Could you check a few things on this drawing? It's one solid part, dimensions in mm from its lowest x, y, z. A direction names the side the tool comes from. Coordinates: 2 decimals unless noted, no trailing zeros. Loops run counter-clockwise (first coordinate to the right, second up) from the corner with the lowest first, then second, coordinate; pieces in that order, holes last.
1) Thinking about a two-plate mould opening in Y: for the marked faces 1, 2 and 3, which applies, released by +Y, released by -Y, zero draft, split by the parting line, or undercut?
2) Imagine slicing it at C-C on y = 3.5. Please give me the cut outline in (x, z), plus the area to 3 significant figures.
3) If I drill on line 1 along Y through (x, z) = (4, 9.25); line 2 along Y through (x, z) = (4, 7.5); line 3 along Y through (x, z) = (4, 11), over which ranges is the centre line in solid material (lowest first)?
4) Imagine slicing it at B-B on x = 4. Please give me the cut outline in (y, z), plus the area to 3 significant figures.
5) Imagine slicing it at A-A on z = 9. Please give me the cut outline in (x, y).
6) Will these pins go through, and if not, where does the flat tip stop? P1, Ø3.5, axis at x = 4, y = 19.5, coming from the -Z side; P2, Ø1.4, axis at x = 4, y = 11, coming from the -Z side; P3, Ø5, axis at y = 9, z = 12, coming from the -X side; P4, Ø1.5, axis at x = 5, z = 6, coming from the -Y side.
7) For the marked faces 4, 5, 6 and 7, which set-ups out of +Z, -Z, +X, -X, +Y, -Y let a thin tool reach every point of the face, with its end or its side?
8) Imagine slicing it at D-D on z = 3.5. Please give me the cut outline in (x, y).
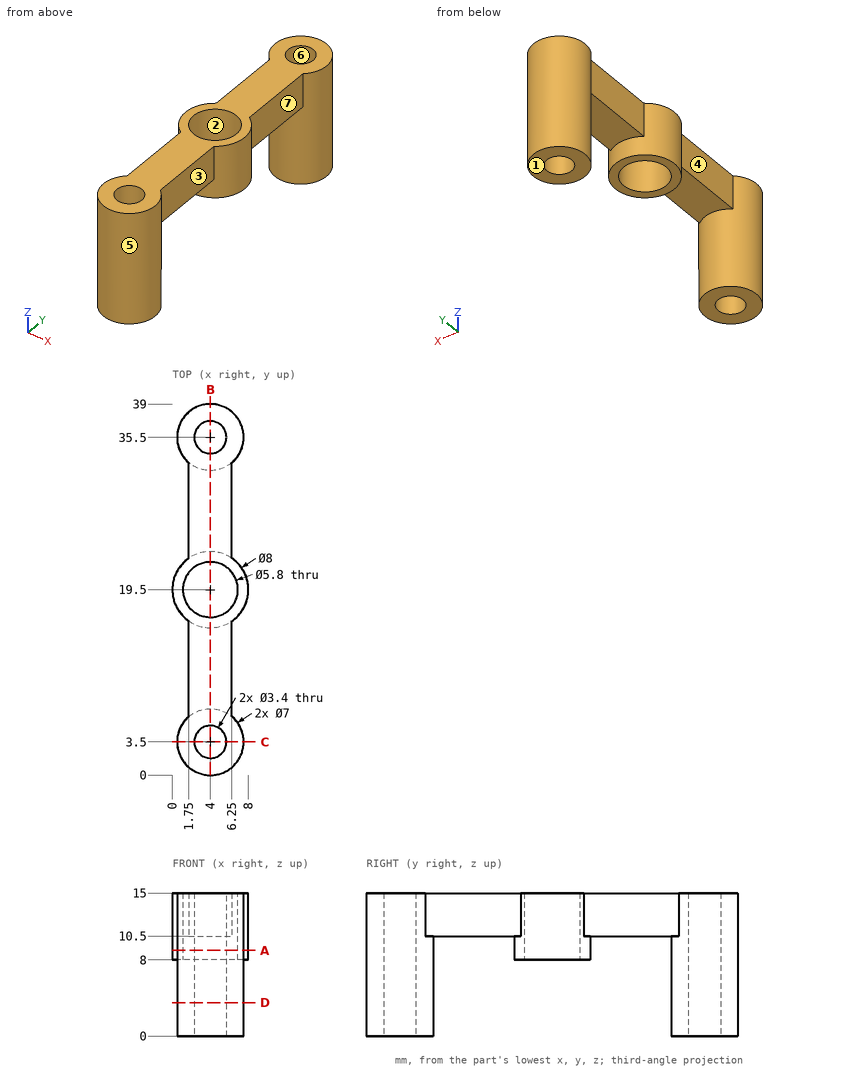
Filled in:
1. face 1: zero draft
1. face 2: undercut
1. face 3: undercut
2. outline: (0.5, 0) - (2.3, 0) - (2.3, 15) - (0.5, 15) - close; (5.7, 0) - (7.5, 0) - (7.5, 15) - (5.7, 15) - close
2. area: 54.0 mm2
3. line 1: y = 0 to 1.8, 5.2 to 7, 15.5 to 16.6, 22.4 to 23.5, 32 to 33.8, 37.2 to 39
3. line 2: y = 0 to 1.8, 5.2 to 7, 32 to 33.8, 37.2 to 39
3. line 3: y = 0 to 1.8, 5.2 to 16.6, 22.4 to 33.8, 37.2 to 39
4. outline: (0, 0) - (1.8, 0) - (1.8, 15) - (0, 15) - close; (5.2, 0) - (7, 0) - (7, 10.5) - (15.5, 10.5) - (15.5, 8) - (16.6, 8) - (16.6, 15) - (5.2, 15) - close; (22.4, 8) - (23.5, 8) - (23.5, 10.5) - (32, 10.5) - (32, 0) - (33.8, 0) - (33.8, 15) - (22.4, 15) - close; (37.2, 0) - (39, 0) - (39, 15) - (37.2, 15) - close
4. area: 200 mm2
5. outline: circle Ø8 at (4, 19.5); circle Ø7 at (4, 3.5); circle Ø7 at (4, 35.5); hole circle Ø5.8 at (4, 19.5); hole circle Ø3.4 at (4, 3.5); hole circle Ø3.4 at (4, 35.5)
6. P1: passes through
6. P2: stops at z = 10.5
6. P3: stops at x = 1.75
6. P4: stops at y = 0.01
7. face 4: +Z, -Z, -X
7. face 5: -Z
7. face 6: +Z, -Z
7. face 7: +Z, -Z, +X
8. outline: circle Ø7 at (4, 3.5); circle Ø7 at (4, 35.5); hole circle Ø3.4 at (4, 3.5); hole circle Ø3.4 at (4, 35.5)
